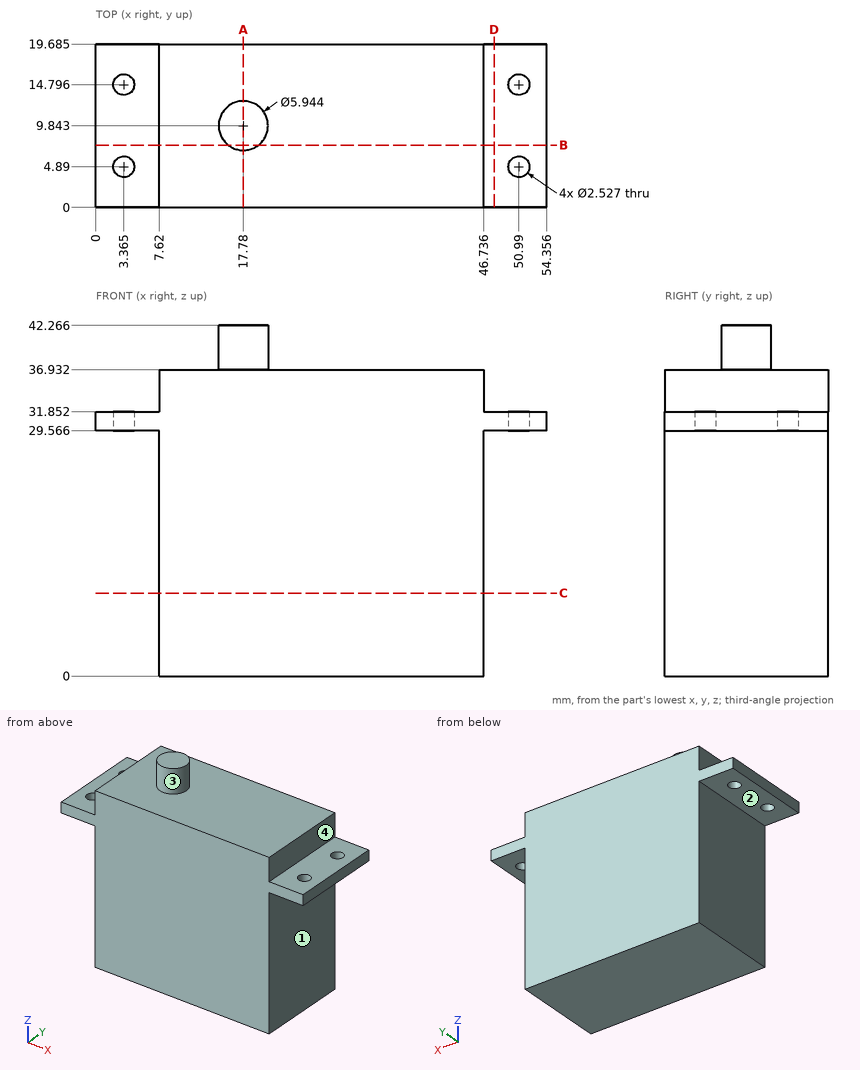
The figure shows three views and two pictorial views of one solid part (mm, origin at its lowest corner). Answer the questions. A direction names the side the tool comes from. Give positions to 0.01 mm unless a question says otherwise; leave off trailing zeros. Write each loop counter-clockwise with the first axis right and the second up, starting at its lowest first coordinate (ties: lowest second). Pieces come first, ordered by that corner, then holes. Notation, with made-up numbers: (33.25, 16) - (62.25, 16) arc R24 ccw to (62.25, 55) - close; hole circle Ø6 at (17.5, 24.5). An arc over 180 degrees is marked (long way). Use one line per item in the form item = value. Start each with the question number.
1) Find section C-C on z = 10. Determine the outline of the cut face in (x, y) (1 decimal).
2) A tool of negligible diameter and unlimited length cuts with its end or side. For the marked faces 1, 2, 3 and 4, from which of +Z, -Z, +X, -X, +Y, -Y can it reach the whole face along a straight path? Write none if from no direction.
3) Find section D-D on x = 48. Determine the outline of the cut face in (y, z) (1 decimal).
4) Find section B-B on y = 7.5. Determine the outline of the cut face in (x, z) (1 decimal), plus the area to 3 significant figures.
5) Find section A-A on x = 17.78. Determine the outline of the cut face in (y, z) (1 decimal), plus the area to 3 significant figures.
6) Consider line 1 along Z through (x, y) = (33, 8.25); line 2 along X through (y, z) = (8.75, 25.5) (1 decimal); line 3 along Z through (x, y) = (52.5, 8.75) (1 decimal). Determine where each line is inside the solid, lowest interval first. Write a range as from..to.
7) Flat-ended cylindrical pins translate along their axes: pin 1 Ø2.5 at (x, y) = (49, 13) entering from -Z; pin 2 Ø2.5 at (y, z) = (13.5, 35) entering from +X; pin 3 Ø3 at (x, y) = (50.99, 4.89) entering from +Z. Find the tip coordinate at first contact, or state that the pin passes through.
Geometry results:
q1.outline = (7.6, 0) - (46.7, 0) - (46.7, 19.7) - (7.6, 19.7) - close
q2.face_1 = -Z, +X, +Y, -Y
q2.face_2 = -Z, -X, +Y, -Y
q2.face_3 = +Z
q2.face_4 = +Z, +X, +Y, -Y
q3.outline = (0, 29.6) - (19.7, 29.6) - (19.7, 31.9) - (0, 31.9) - close
q4.outline = (0, 29.6) - (7.6, 29.6) - (7.6, 0) - (46.7, 0) - (46.7, 29.6) - (54.4, 29.6) - (54.4, 31.9) - (46.7, 31.9) - (46.7, 36.9) - (19.6, 36.9) - (19.6, 42.3) - (16, 42.3) - (16, 36.9) - (7.6, 36.9) - (7.6, 31.9) - (0, 31.9) - close
q4.area = 1,500 mm2
q5.outline = (0, 0) - (19.7, 0) - (19.7, 36.9) - (12.8, 36.9) - (12.8, 42.3) - (6.9, 42.3) - (6.9, 36.9) - (0, 36.9) - close
q5.area = 759 mm2
q6.line_1 = 0..36.93
q6.line_2 = 7.6..46.7
q6.line_3 = 29.6..31.9
q7.pin_1 = 29.57
q7.pin_2 = 46.74
q7.pin_3 = 31.85
